Part model, mm, in its own coordinate system. A direction names the side the tool comes from. Round coordinates to 2 decimals unless told otherwise and drop trailing zeros. Loops run counter-clockwise (first coordinate to the right, second up) from the corner with the lowest first, then second, coordinate; pieces in that order, holes last.
1) Mould opens along Z. For faces 1 (the flat face through (7.5, 1, 0)), 2 (the flat face through (0, 2, -3.5)), 3 (the cylindrical face through (0.02, 4.56, 0.54)) say: +Z half, -Z half, draft (parallel to the pull), parting line (faces both ways), or undercut.
2) Band-saw the part on C-C, the plane z = 0. Write the cut outline in (x, y).
3) 3-axis set-ups, long thin cutter, end or side, ignore diameter. For faces 4 (the flat face through (0, 12, 0)), 5 (the flat face through (1.5, 5, -2)), 6 (the flat face through (-6, 2, -1)): which of +Z, -Z, +X, -X, +Y, -Y reach the whole face in a straight line?
4) Probe line 1 (X direction, y = 0.8, z = 0); line 2 (X direction, y = 2.25, z = 3.25); line 3 (Y direction, x = 6.25, z = 1). List the from-to ranges inside material, lowest first.
5) Band-saw the part on B-B, the plane x = -4.5. Write the cut outline in (y, z), then the cut area to 3 significant figures.
6) Band-saw the part on A-A, the plane y = 7. Write the cut outline in (x, z), then the cut area to 3 significant figures.
7) Band-saw the part on D-D, the plane y = 1.75. Write the cut outline in (x, z).
8) Drop flat-ended pins along their axis: P1, Ø1.5, axis at y = 4.5, z = 0.5, coming from the +X side; P2, Ø1.5, axis at x = -4.5, z = -2.5, coming from the +Y side; P3, Ø2, axis at y = 10, z = -0.5, coming from the -X side. Give the stop position or say it passes through.
from build123d import *

# Parameters (mm, degrees)
SKETCH1_W           = 15
SKETCH1_H           = 7
BOSS_EXTRUDE1_DEPTH = 2
SKETCH2_W           = 3
SKETCH2_H           = 7
BOSS_EXTRUDE2_DEPTH = 10
SKETCH3_R           = 2.5
CUT_EXTRUDE1_DEPTH  = 10
FILLET1_R           = 3
SKETCH4_R           = 1.5
CUT_EXTRUDE2_DEPTH  = 10


with BuildPart() as part:
    # Sketch1 → Boss-Extrude1 (new body)
    with BuildSketch(Plane(origin=(0, 0, 0), x_dir=(1, 0, 0), z_dir=(0, 1, 0))):
        Rectangle(SKETCH1_W, SKETCH1_H)
    extrude(amount=BOSS_EXTRUDE1_DEPTH)

    # Sketch2 → Boss-Extrude2 (add)
    with BuildSketch(Plane(origin=(0, 2, 0), x_dir=(1, 0, 0), z_dir=(0, 1, 0))):
        Rectangle(SKETCH2_W, SKETCH2_H)
    extrude(amount=BOSS_EXTRUDE2_DEPTH)

    # Sketch3 → Cut-Extrude1 (cut)
    with BuildSketch(Plane(origin=(1.5, 0, 0), x_dir=(0, 0, -1), z_dir=(1, 0, 0))):
        with Locations((0, 7)):
            Circle(SKETCH3_R)
    extrude(amount=-CUT_EXTRUDE1_DEPTH, mode=Mode.SUBTRACT)

    # Fillet1
    fillet1_edges = [part.edges().sort_by_distance(p)[0] for p in [
        (0, 12, 3.5),
        (0, 12, -3.5),
    ]]
    fillet(fillet1_edges, radius=FILLET1_R)

    # Sketch4 → Cut-Extrude2 (cut)
    with BuildSketch(Plane(origin=(0, 2, 0), x_dir=(1, 0, 0), z_dir=(0, 1, 0))):
        with Locations(Location((4.5, 0, 0), (0, 0, 270))):
            Circle(SKETCH4_R)
        with Locations(Location((-4.5, 0, 0), (0, 0, 270))):
            Circle(SKETCH4_R)
    extrude(amount=-CUT_EXTRUDE2_DEPTH, mode=Mode.SUBTRACT)


solid = part.part
Reported:
1. face 1: draft
1. face 2: -Z half
1. face 3: undercut
2. outline: (-7.5, 0) - (-6, 0) - (-6, 2) - (-7.5, 2) - close; (-3, 0) - (3, 0) - (3, 2) - (1.5, 2) - (1.5, 4.5) - (-1.5, 4.5) - (-1.5, 2) - (-3, 2) - close; (-1.5, 9.5) - (1.5, 9.5) - (1.5, 12) - (-1.5, 12) - close; (6, 0) - (7.5, 0) - (7.5, 2) - (6, 2) - close
3. face 4: +Z, -Z, +X, -X, +Y
3. face 5: +Z, -Z, +X, +Y
3. face 6: +Z, -Z, -X, +Y
4. line 1: x = -7.5 to -6, -3 to 3, 6 to 7.5
4. line 2: x = -1.5 to 1.5
4. line 3: y = 0 to 2
5. outline: (0, -3.5) - (2, -3.5) - (2, -1.5) - (0, -1.5) - close; (0, 1.5) - (2, 1.5) - (2, 3.5) - (0, 3.5) - close
5. area: 8.00 mm2
6. outline: (-1.5, -3.5) - (1.5, -3.5) - (1.5, -2.5) - (-1.5, -2.5) - close; (-1.5, 2.5) - (1.5, 2.5) - (1.5, 3.5) - (-1.5, 3.5) - close
6. area: 6.00 mm2
7. outline: (-7.5, -3.5) - (7.5, -3.5) - (7.5, 3.5) - (-7.5, 3.5) - close; hole circle Ø3 at (-4.5, 0); hole circle Ø3 at (4.5, 0)
8. P1: stops at x = 1.5
8. P2: stops at y = 2
8. P3: stops at x = -1.5
